Part model, mm, in its own coordinate system. Face numbers are marked on the shaded views. A direction names the side the tool comes from. Coordinates: 2 decimals unless noted, no trailing zeros. Loops run counter-clockwise (first coordinate to the right, second up) from the corner with the lowest first, then second, coordinate; pieces in that order, holes last. Notation, with made-up numbers: (-32, -35) -> (20, -35) arc R20 cw to (20, -29) -> close; hole circle Ø2 at (16.25, 0). An arc over 180 degrees is marked (long way). One line per item, written item: value. Start each with the question number.
from build123d import *

# Parameters (mm, degrees)
F0_R     = 118.3690263596
F1_DEPTH = 177.8
F2_R     = 37.4516479343
F3_DEPTH = 203.2
F5_DEPTH = 38.1


with BuildPart() as f1:
    # F0 (on Top) → F1 (new body)
    with BuildSketch(Plane.XY):
        Circle(F0_R)
    extrude(amount=F1_DEPTH)

    # F2 (on face) → F3 (join)
    with BuildSketch(Plane.XY.offset(177.8)):
        Circle(F2_R)
    extrude(amount=F3_DEPTH)

    # F4 (on face) → F5 (join)
    with BuildSketch(Plane.XY.offset(381)):
        with BuildLine():
            Line((27.6787410495, 25.2292137593), (0, 25.2292137593))
            Line((0, 25.2292137593), (-27.6787410495, 25.2292137593))
            ThreePointArc((-27.6787410495, 25.2292137593), (-37.0697451311, -5.3347848045), (-19.441274734, -32.0103541017))
            Line((-19.441274734, -32.0103541017), (0, -32.0103541017))
            Line((0, -32.0103541017), (19.441274734, -32.0103541017))
            ThreePointArc((19.441274734, -32.0103541017), (32.6399579483, -18.3646148376), (37.4516479343, 0))
            ThreePointArc((37.4516479343, 0), (34.9230611348, 13.5279611906), (27.6787410495, 25.2292137593))
        make_face()
        with BuildLine():
            Line((83.6336314678, 25.2292137593), (27.6787410495, 25.2292137593))
            ThreePointArc((27.6787410495, 25.2292137593), (34.9230611348, 13.5279611906), (37.4516479343, 0))
            ThreePointArc((37.4516479343, 0), (32.6399579483, -18.3646148376), (19.441274734, -32.0103541017))
            Line((19.441274734, -32.0103541017), (83.6336314678, -32.0103541017))
            Line((83.6336314678, -32.0103541017), (83.6336314678, 0))
            Line((83.6336314678, 0), (83.6336314678, 25.2292137593))
        make_face()
        with BuildLine():
            ThreePointArc((-19.441274734, -32.0103541017), (-37.0697451311, -5.3347848045), (-27.6787410495, 25.2292137593))
            Line((-27.6787410495, 25.2292137593), (-207.8490108252, 25.2292137593))
            Line((-207.8490108252, 25.2292137593), (-207.8490108252, 0))
            Line((-207.8490108252, 0), (-207.8490108252, -32.0103541017))
            Line((-207.8490108252, -32.0103541017), (-19.441274734, -32.0103541017))
        make_face()
    extrude(amount=F5_DEPTH)


solid = f1.part
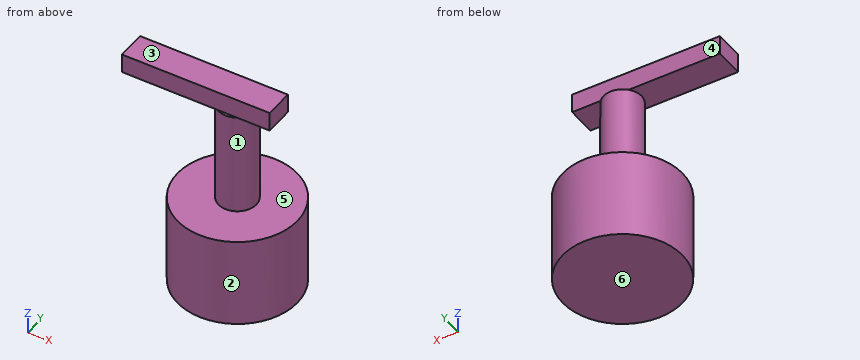
1) Probe line 1 (Z direction, x = -98, y = 8.5); line 2 (Y direction, x = -142.5, z = 401); line 3 (X direction, y = -18.5, z = 398.5). List the from-to ranges inside material, lowest first. Write a range as from..to.
2) Pin check, flat tips, straight feed: pin 1 Ø3 at (x, z) = (-31.5, 158) entering from +Y; pin 2 Ø5 at (x, z) = (24, 211.5) entering from -Y; pin 3 Ø6 at (x, y) = (-6.5, -36) entering from +Z. Stop position of each tip, or through.
3) Slice it at B-B (y = 0). Give the cut face in (x, z).
4) Slice it at C-C (x = 0). Give the cut face in (y, z), then the cut area to 3 significant figures.
5) Slice it at A-A (x = 70). Give the cut face in (y, z), then the cut area to 3 significant figures.
6) Tool access for the marked faces 4, 5 and 6: list every direction of +Z, -Z, +X, -X, +Y, -Y with a clear straight run to the whole face (end or side of a thin tool).
7) Pull direction Z, two halves, no side cores. Call the marked faces 1, 2 and 3: +Z half, -Z half, draft (parallel to the pull), parting line (faces both ways), or undercut.
8) Slice it at D-D (z = 77). Give the cut face in (x, y), then the cut area to 3 significant figures.
Check sheet entries:
1. line 1: z = 0..177.8, 381..419.1
1. line 2: y = -32.01..25.23
1. line 3: x = -207.85..83.63
2. pin 1: stops at y = 114.5
2. pin 2: stops at y = -30.67
2. pin 3: stops at z = 381
3. outline: (-207.85, 381) -> (-37.45, 381) -> (-37.45, 177.8) -> (-118.37, 177.8) -> (-118.37, 0) -> (118.37, 0) -> (118.37, 177.8) -> (37.45, 177.8) -> (37.45, 381) -> (83.63, 381) -> (83.63, 419.1) -> (-207.85, 419.1) -> close
4. outline: (-118.37, 0) -> (118.37, 0) -> (118.37, 177.8) -> (37.45, 177.8) -> (37.45, 381) -> (25.23, 381) -> (25.23, 419.1) -> (-32.01, 419.1) -> (-32.01, 381) -> (-37.45, 381) -> (-37.45, 177.8) -> (-118.37, 177.8) -> close
4. area: 59,500 mm^2
5. outline: (-95.45, 0) -> (95.45, 0) -> (95.45, 177.8) -> (-95.45, 177.8) -> close; (-32.01, 381) -> (25.23, 381) -> (25.23, 419.1) -> (-32.01, 419.1) -> close
5. area: 36,100 mm^2
6. face 4: +Z, +X, -X, +Y
6. face 5: none
6. face 6: -Z, +X, -X, +Y, -Y
7. face 1: undercut
7. face 2: draft
7. face 3: +Z half
8. outline: circle Ø236.74 at (0, 0)
8. area: 44,000 mm^2
